Design review of the part built by this model. Coordinates are the model's own, in mm. A direction names the side the tool comes from. Give positions to 0.01 mm unless a question says otherwise; leave off trailing zeros. Loops run counter-clockwise (first coordinate to the right, second up) from the corner with the lowest first, then second, coordinate; pieces in that order, holes last. Notation, with made-up numbers: (46.25, 0) -> (82.25, 0) arc R21 cw to (82.25, 27) -> close; hole circle Ø3 at (21.25, 20). An arc over 180 degrees is marked (long way). Answer as CSV lines item,"result".
from build123d import *

# Parameters (mm, degrees)
EXTRUDE_1_DEPTH                  = 40
EXTRUDE_1_DEPTH_BACK             = 4
SKETCH_1_R                       = 46
EXTRUDE_START                    = -4
SKETCH_2_R                       = 8
EXTRUDE_2_DEPTH                  = 44
FILLET_1_R                       = 10
PATTERN_CIRCULAR_1_COUNT         = 3
FILLET_1_OF_PATTERN_CIRCULAR_1_R = 10
EXTRUDE_3_DEPTH                  = 52
EXTRUDE_4_DEPTH                  = 9
EXTRUDE_5_DEPTH                  = 20
FILLET_2_R                       = 20
FILLET_3_R                       = 5
RIB_1_REACH                      = 166.697
SKETCH_6_WALL_W                  = 367.279305732
SKETCH_6_WALL_H                  = 9
EXTRUDE_6_DEPTH                  = 64
EXTRUDE_6_DEPTH_BACK             = 11
SKETCH_8_W                       = 116
SKETCH_8_H                       = 11
CUT_EXTRUDE_1_DEPTH              = 64
SKETCH_9_R                       = 36
SKETCH_9_R_2                     = 3.5
CUT_EXTRUDE_2_DEPTH              = 64
HOLE_WIZARD_M10_1_REACH          = 239.276
HOLE_WIZARD_M10_1_BORE_R         = 4.25


with BuildPart() as part:
    # 草图1 → 凸台-拉伸1 (new, two sides: drawn at the far end of the back side and taken through both)
    with BuildSketch(Plane.XY.offset(-EXTRUDE_1_DEPTH_BACK)):
        Circle(SKETCH_1_R)
    extrude(amount=EXTRUDE_1_DEPTH + EXTRUDE_1_DEPTH_BACK)

    # 草图2 → 凸台-拉伸2 (add)
    with BuildSketch(Plane.XY.offset(EXTRUDE_START)):
        with Locations((0, -46)):
            Circle(SKETCH_2_R)
    extrude_2 = extrude(amount=EXTRUDE_2_DEPTH)

    # 圆角1
    fillet_1_edges = [part.edges().sort_by_distance(p)[0] for p in [
        (7.969696861, -45.304347826, 18),
        (-7.969696861, -45.304347826, 18),
    ]]
    fillet(fillet_1_edges, radius=FILLET_1_R)

    # 阵列(圆周)1: 凸台-拉伸2 ×3 about axis
    pattern_circular_1_axis = Axis((0, 0, 0), (0, 0, 1))
    for i in range(1, PATTERN_CIRCULAR_1_COUNT):
        add(extrude_2.rotate(pattern_circular_1_axis, i * 360 / PATTERN_CIRCULAR_1_COUNT))

    # 圆角1 of 阵列(圆周)1
    fillet_1_of_pattern_circular_1_edges = [part.edges().sort_by_distance(p)[0] for p in [
        (35.249867689, 29.554133855, 18),
        (43.21956455, 15.750213971, 18),
        (-43.21956455, 15.750213971, 18),
        (-35.249867689, 29.554133855, 18),
    ]]
    fillet(fillet_1_of_pattern_circular_1_edges, radius=FILLET_1_OF_PATTERN_CIRCULAR_1_R)

    # 草图3 → 凸台-拉伸3 (add)
    with BuildSketch(Plane(origin=(0, 0, 0), x_dir=(1, 0, 0), z_dir=(0, 1, 0))):
        with BuildLine():
            Line((-12, 4), (12, 4))
            Line((12, 4), (12, -18))
            ThreePointArc((12, -18), (0, -30), (-12, -18))
            Line((-12, -18), (-12, 4))
        make_face()
    extrude(amount=EXTRUDE_3_DEPTH)

    # 草图4 → 凸台-拉伸4 (add)
    with BuildSketch(Plane.XY):
        Polygon((-55, -150), (55, -150), (41, -20.856653615), (-41, -20.856653615), align=None)
    extrude(amount=EXTRUDE_4_DEPTH)

    # 草图5 → 凸台-拉伸5 (add)
    with BuildSketch(Plane.XY.offset(9)):
        Polygon((-41, -20.856653615), (-55, -150), (-45.947270441, -150), (-32.052422425, -21.826630695), align=None)
    extrude_5 = extrude(amount=EXTRUDE_5_DEPTH)

    # 镜向1: 凸台-拉伸5 across plane
    add(extrude_5.mirror(Plane(origin=(0, 0, 0), x_dir=(0, 0, 1), z_dir=(1, 0, 0))))

    # 圆角2
    fillet_2_edges = [part.edges().sort_by_distance(p)[0] for p in [
        (41, -20.856653615, 14.5),
        (-41, -20.856653615, 14.5),
    ]]
    fillet(fillet_2_edges, radius=FILLET_2_R)

    # 圆角3
    fillet_3_edges = [part.edges().sort_by_distance(p)[0] for p in [
        (-33.144192236, -31.897688333, 19),
        (33.144192236, -31.897688333, 19),
    ]]
    fillet(fillet_3_edges, radius=FILLET_3_R)

    # 草图6 wall → 筋1 (add, up to next)
    with BuildSketch(Plane(origin=(0, -68, 18.777260671), x_dir=(0, -0.780250226157, -0.625467492826), z_dir=(0, 0.625467492826, -0.780250226157)), mode=Mode.PRIVATE) as rib_1_sk1:
        Rectangle(SKETCH_6_WALL_W, SKETCH_6_WALL_H)
    rib_1_tool1 = extrude(rib_1_sk1.sketch, amount=RIB_1_REACH, mode=Mode.PRIVATE) - part.part
    add(rib_1_tool1.solids().sort_by_distance((0, -68, 18.777260671))[0])

    # 草图7 → 凸台-拉伸6 (add, two sides: drawn at the far end of the back side and taken through both)
    with BuildSketch(Plane.XY.offset(-EXTRUDE_6_DEPTH_BACK)):
        Polygon((-70, -150), (70, -150), (70, -170), (58, -170), (58, -164), (6, -164), (6, -170), (-6, -170), (-6, -164), (-58, -164), (-58, -170), (-70, -170), align=None)
    extrude(amount=EXTRUDE_6_DEPTH + EXTRUDE_6_DEPTH_BACK)

    # 草图8 → 切除-拉伸1 (cut)
    with BuildSketch(Plane(origin=(0, -150, 0), x_dir=(1, 0, 0), z_dir=(0, 1, 0))):
        with Locations((0, 5.5)):
            Rectangle(SKETCH_8_W, SKETCH_8_H)
        with BuildLine():
            Line((-43, -40), (-43, -64))
            Line((-43, -64), (-27, -64))
            Line((-27, -64), (-27, -40))
            ThreePointArc((-27, -40), (-35, -32), (-43, -40))
        make_face()
        with BuildLine():
            Line((43, -40), (43, -64))
            Line((43, -64), (27, -64))
            Line((27, -64), (27, -40))
            ThreePointArc((27, -40), (35, -32), (43, -40))
        make_face()
    extrude(amount=-CUT_EXTRUDE_1_DEPTH, mode=Mode.SUBTRACT)

    # 草图9 → 切除-拉伸2 (cut)
    with BuildSketch(Plane.XY.offset(40)):
        Circle(SKETCH_9_R)
        with Locations((-39.837168574, 23)):
            Circle(SKETCH_9_R_2)
        with Locations((39.837168574, 23)):
            Circle(SKETCH_9_R_2)
        with Locations((0, -46)):
            Circle(SKETCH_9_R_2)
    extrude(amount=-CUT_EXTRUDE_2_DEPTH, mode=Mode.SUBTRACT)

    # M10 螺纹孔1 bore (on position points) → M10 螺纹孔1 (cut, up to next)
    with BuildSketch(Plane(origin=(0, 52, 18), x_dir=(0, 0, 1), z_dir=(0, 1, 0)), mode=Mode.PRIVATE) as hole_wizard_m10_1_sk1:
        Circle(HOLE_WIZARD_M10_1_BORE_R)
    hole_wizard_m10_1_tool1 = extrude(hole_wizard_m10_1_sk1.sketch, amount=-HOLE_WIZARD_M10_1_REACH, mode=Mode.PRIVATE) & part.part
    add(hole_wizard_m10_1_tool1.solids().sort_by_distance((0, 52, 18))[0], mode=Mode.SUBTRACT)


solid = part.part
Q1. We need section D-D, the plane x = -50.5. State the section outline as (y, z) points.
Filled sheet:
outline,"(-164, 0) -> (-108.49, 0) -> (-108.49, 29) -> (-150, 29) -> (-150, 64) -> (-164, 64) -> close"
Q2. We need section C-C, the plane y = -117. State the section outline as (x, z) points, and give its area (3 significant figures).
Filled sheet:
outline,"(-51.42, 0) -> (51.42, 0) -> (51.42, 29) -> (42.37, 29) -> (42.37, 9) -> (-42.37, 9) -> (-42.37, 29) -> (-51.42, 29) -> close"
area,"1,290 mm^2"
Q3. Clearance check with flat-ended pins moving along their axes: pin 1 Ø10 at (x, z) = (-27, 53.5) entering from +Y; pin 2 Ø1.5 at (x, y) = (-27, -114.5) entering from +Z; pin 3 Ø3 at (x, z) = (-26.5, 33.5) entering from -Y; pin 4 Ø6.5 at (x, y) = (0, -46) entering from +Z. State where each tip first meets the part, or that it passes through.
Filled sheet:
pin 1,"stops at y = -150"
pin 2,"stops at z = 9"
pin 3,"stops at y = -164"
pin 4,"passes through"
Q4. The part is to be moulded in two halves that separate along Y. For faces 6 (the flat face through (-43, -157, 52)), 7 (the flat face through (40.137, -96.402, 18.86)), 8 (the cylindrical face through (8.12, 45.278, 27.47)), say which applies: pulls with the +Y half, pulls with the -Y half, needs draft (parallel to the pull), parting line crosses it, or undercut.
Filled sheet:
face 6,"needs draft"
face 7,"undercut"
face 8,"pulls with the +Y half"
Q5. To check wall thickness, follow probe 1 along X at (y, z) = (1.5, 33); probe 2 along X at (y, z) = (46.5, 18); probe 3 along X at (y, z) = (25.5, 6). State the ranges of each line that lie inside material, in increasing order. Write a range as from..to.
Filled sheet:
probe 1,"x = -45.98..-35.97, 35.97..45.98"
probe 2,"x = -12..-4.25, 4.25..12"
probe 3,"x = -47.44..-42.29, -37.39..-25.41, 25.41..37.39, 42.29..47.44"
Q6. For faces 1 (the flat face through (-40.137, -96.402, 18.86)), 2 (the flat face through (-12, 48, 7)), 3 (the flat face through (64, -160, -11)), 4 (the flat face through (-27, -157, 52)), 5 (the flat face through (-48.196, -87.235, 14.297)), list the 3-axis set-ups (+Z, -Z, +X, -X, +Y, -Y) from which the entire face can be reached by the end or side of a thin tool; tool diameter is ignored.
Filled sheet:
face 1,"+Z"
face 2,"+Z, -Z, -X, +Y"
face 3,"-Z, +X, -X, +Y, -Y"
face 4,"+Z, +Y, -Y"
face 5,"+Z, -Z, -X"
Q7. We need section B-B, the plane y = 23. State the section outline as (x, z) points, and give its area (3 significant figures).
Filled sheet:
outline,"(-47.84, -4) -> (-43.34, -4) -> (-43.34, 40) -> (-47.84, 40) -> close; (-36.34, -4) -> (-27.69, -4) -> (-27.69, 40) -> (-36.34, 40) -> close; (27.69, -4) -> (36.34, -4) -> (36.34, 40) -> (27.69, 40) -> close; (43.34, -4) -> (47.84, -4) -> (47.84, 40) -> (43.34, 40) -> close"
area,"1,160 mm^2"
Q8. We need section A-A, the plane z = 54.5. State the section outline as (x, y) points.
Filled sheet:
outline,"(-70, -170) -> (-58, -170) -> (-58, -164) -> (-43, -164) -> (-43, -150) -> (-70, -150) -> close; (-27, -164) -> (-6, -164) -> (-6, -170) -> (6, -170) -> (6, -164) -> (27, -164) -> (27, -150) -> (-27, -150) -> close; (43, -164) -> (58, -164) -> (58, -170) -> (70, -170) -> (70, -150) -> (43, -150) -> close"
